from build123d import *

# Parameters (mm, degrees)
CROQUIS1_R              = 1.1
SALIENTE_EXTRUIR1_DEPTH = 1.7
CROQUIS2_R              = 3.5
CROQUIS2_R_2            = 2.4
SALIENTE_EXTRUIR2_DEPTH = 3
CROQUIS3_R              = 2.25
CORTAR_EXTRUIR1_DEPTH   = 1


with BuildPart() as part:
    # Croquis1 → Saliente-Extruir1 (new body)
    with BuildSketch(Plane.XY):
        with BuildLine():
            ThreePointArc((1.75, 15), (0, 16.75), (-1.75, 15))
            Line((-1.75, 15), (-3.406001644, 0.805700192))
            Line((-3.406001644, 0.805700192), (-3.5, 0))
            ThreePointArc((-3.5, 0), (0, -3.5), (3.5, 0))
            Line((3.5, 0), (3.406001644, 0.805700192))
            Line((3.406001644, 0.805700192), (1.75, 15))
        make_face()
        Circle(CROQUIS1_R, mode=Mode.SUBTRACT)
        with BuildLine():
            ThreePointArc((-0.7, 15), (0, 15.7), (0.7, 15))
            Line((0.7, 15), (0.7, 4.5))
            ThreePointArc((0.7, 4.5), (0, 3.8), (-0.7, 4.5))
            Line((-0.7, 4.5), (-0.7, 15))
        make_face(mode=Mode.SUBTRACT)
    extrude(amount=SALIENTE_EXTRUIR1_DEPTH)

    # Croquis2 → Saliente-Extruir2 (add)
    with BuildSketch(Plane.XY.offset(1.7)):
        Circle(CROQUIS2_R)
        Circle(CROQUIS2_R_2, mode=Mode.SUBTRACT)
    extrude(amount=SALIENTE_EXTRUIR2_DEPTH)

    # Croquis3 → Cortar-Extruir1 (cut)
    with BuildSketch(Plane(origin=(0, 0, 0), x_dir=(-1, 0, 0), z_dir=(0, 0, -1))):
        Circle(CROQUIS3_R)
    extrude(amount=-CORTAR_EXTRUIR1_DEPTH, mode=Mode.SUBTRACT)


solid = part.part
CAD build for the part. Positions are in the model's coordinates, mm. A direction names the side the tool comes from. Round coordinates to 2 decimals unless told otherwise and drop trailing zeros. Order: outer loops, then holes, each group sorted by start corner. A loop starts at its lowest first (then second) coordinate and runs counter-clockwise, first axis right, second up. Notation, with made-up numbers: (18.5, -30) -> (75.5, -30) arc R20 ccw to (75.5, -14) -> close; hole circle Ø10 at (29, 6). An arc over 180 degrees is marked (long way). Write item = value, one per line. Start each with the question number.
(1) Cut at D-D, the plane z = 3.8. List the corners of the cut face in (x, y).
(2) Cut at C-C, the plane y = 13. List the corners of the cut face in (x, z), then the cut area to 3 significant figures.
(3) Which spindle directions (+Z, -Z, +X, -X, +Y, -Y) get a long thin tool onto all of the face, cutting with end or side? Do faces 1 (the flat face through (1, 7, 0)), 2 (the cylindrical face through (0.29, 2.23, 0.49)), 3 (the flat face through (0.7, 10, 1)), 4 (the cylindrical face through (1.29, 2.024, 3.179)). Say none if no direction does.
(4) Pin check, flat tips, straight feed: P1, Ø2.5, axis at x = 0, y = 0, coming from the +Z side; P2, Ø1.3, axis at x = 0, y = 0.5, coming from the -Z side; P3, Ø0.8, axis at y = 9.5, z = 1, coming from the -X side. Stop position of each tip, or through.
(5) Pull direction Y, two halves, no side cores. Call faces 5 (the cylindrical face through (0.04, 16.75, 0.84)), 6 (the flat face through (-1, 9, 1.7)), 7 (the cylindrical face through (0, 3.8, 0.8)): released by +Y, released by -Y, zero draft, split by the parting line, or undercut.
(6) Probe line 1 (Y direction, x = 0, z = 1.3); line 2 (Y direction, x = 0, z = 3.85); line 3 (X direction, y = 15, z = 1.3). List the from-to ranges inside material, lowest first. Write a range as [from, to].
(7) Cut at B-B, the plane z = 1.45. List the corners of the cut face in (x, y), then the cut area to 3 significant figures.
Model answer:
q1.outline = circle Ø7 at (0, 0); hole circle Ø4.8 at (0, 0)
q2.outline = (-1.98, 0) -> (-0.7, 0) -> (-0.7, 1.7) -> (-1.98, 1.7) -> close; (0.7, 0) -> (1.98, 0) -> (1.98, 1.7) -> (0.7, 1.7) -> close
q2.area = 4.36 mm2
q3.face_1 = -Z, +X, -X, +Y, -Y
q3.face_2 = -Z
q3.face_3 = +Z, -Z
q3.face_4 = +Z
q4.P1 = 1.7
q4.P2 = 1
q4.P3 = -2.44
q5.face_5 = released by +Y
q5.face_6 = zero draft
q5.face_7 = undercut
q6.line_1 = [-3.5, -1.1], [1.1, 3.8], [15.7, 16.75]
q6.line_2 = [-3.5, -2.4], [2.4, 3.5]
q6.line_3 = [-1.75, -0.7], [0.7, 1.75]
q7.outline = (-3.5, 0) arc R3.5 ccw to (3.5, 0) -> (1.75, 15) arc R1.75 ccw to (-1.75, 15) -> close; hole circle Ø2.2 at (0, 0); hole (-0.7, 4.5) arc R0.7 ccw to (0.7, 4.5) -> (0.7, 15) arc R0.7 ccw to (-0.7, 15) -> close
q7.area = 82.8 mm2
